Geometry: final body of the model. Coordinates: model frame, mm. A direction names the side the tool comes from. Round coordinates to 2 decimals unless told otherwise and drop trailing zeros. Write each loop counter-clockwise with the first axis right and the second up, starting at its lowest first coordinate (ties: lowest second). Pieces come first, ordered by that corner, then holes. Notation, with made-up numbers: (-26, -20.75) - (-17, -20.75) arc R23 ccw to (-17, -6.75) - close; hole circle Ø2 at (47.25, 10). An arc over 180 degrees is marked (long way). Write each question's results on one line, items separated by ' | '.
from build123d import *

# Parameters (mm, degrees)
F0_W     = 355.6
F0_H     = 101.6
F1_DEPTH = 9.525
F2_DEPTH = 3.175
F3_W     = 12.7
F3_H     = 6.35
F4_DEPTH = 12.7


# Not quite as in the source:
# - a feature names something its author has since deleted; it is built from what else it names


with BuildPart() as f1:
    # F0 (on Right) → F1 (new body, symmetric)
    with BuildSketch(Plane.YZ):
        with Locations((0, -50.8)):
            Rectangle(F0_W, F0_H)
    extrude(amount=F1_DEPTH, both=True)

    # F0 (on Right) → F2 (join, symmetric)
    with BuildSketch(Plane.YZ):
        Polygon((-177.8, -101.6), (-177.8, 0), (-184.15, 0), (-184.15, -12.7), (-206.375, -12.7), (-206.375, -101.6), align=None)
        Polygon((184.15, 0), (177.8, 0), (177.8, -101.6), (206.375, -101.6), (206.375, -12.7), (184.15, -12.7), align=None)
    extrude(amount=F2_DEPTH, both=True)

    # F3 (on face) → F4 (cut)
    with BuildSketch(Plane.YZ.offset(9.525)):
        with Locations((-165.1, -92.075)):
            Rectangle(F3_W, F3_H)
        with Locations((165.1, -92.075)):
            Rectangle(F3_W, F3_H)
    extrude(amount=-F4_DEPTH, mode=Mode.SUBTRACT)


solid = f1.part
Q1. Section query A-A, the plane z = -44.5. Return loops of the section in (x, y) (3 decimals), plus the area to 3 significant figures.
Answer block:
outline: (-9.525, -177.8) - (-3.175, -177.8) - (-3.175, -206.375) - (3.175, -206.375) - (3.175, -177.8) - (9.525, -177.8) - (9.525, 177.8) - (3.175, 177.8) - (3.175, 206.375) - (-3.175, 206.375) - (-3.175, 177.8) - (-9.525, 177.8) - close | area: 7,140 mm2
Q2. Ray query, line 1 along Y through (x, z) = (-6.5, -87.5); line 2 along Z through (x, y) = (-2.75, 160). Return the intervals inside material, ascending.
Answer block:
line 1: -177.8 to 177.8 | line 2: -101.6 to -95.25, -88.9 to 0
Q3. Pin query (flat end, axial travel): pin 1 (6 mm diameter, centred on x = -7.5, z = -39.5, fed in from +Y); pin 2 (3 mm diameter, centred on x = 7.5, z = -46.5, fed in from -Y); pin 3 (5 mm diameter, centred on x = -0.5, z = -4, fed in from +Y). Return the tip coordinate at first contact, or that it passes through.
Answer block:
pin 1: y = 177.8 | pin 2: y = -177.8 | pin 3: y = 184.15
Q4. Mould query, pull axis Z, two halves, no side actions, for faces 6 (the flat face through (3, 165, -95.25)), 7 (the flat face through (3, 165, -88.9)), 8 (the flat face through (3.175, 192, -50)), 9 (the flat face through (0, -3, -101.6)). Classes: pulls with the +Z half, pulls with the -Z half, needs draft (parallel to the pull), parting line crosses it, or undercut.
Answer block:
face 6: undercut | face 7: undercut | face 8: needs draft | face 9: pulls with the -Z half
Q5. Access query for faces 1 (the flat face through (-3.175, 192, -50)), 2 (the flat face through (3.175, -192, -50)), 3 (the flat face through (3, -165, -95.25)), 4 (the flat face through (-9.525, -2, -50)), 5 (the flat face through (-3.175, -192, -50)). Directions: +Z, -Z, +X, -X, +Y, -Y. A direction counts if a zero-diameter tool reaches every point of the face in a straight line with its end or side. Return the directions, or none.
Answer block:
face 1: +Z, -Z, -X, +Y | face 2: +Z, -Z, +X, -Y | face 3: +X | face 4: +Z, -Z, -X, +Y, -Y | face 5: +Z, -Z, -X, -Y
